Can you work these out from the model? Positions are in its coordinate system, mm. A direction names the side the tool comes from. Coordinates: 2 decimals unless noted, no trailing zeros. Loops run counter-clockwise (first coordinate to the right, second up) from the corner with the lowest first, then second, coordinate; pieces in that order, holes last. Notation, with made-up numbers: M 18,29 L 37,29 A9 cw 37,34 Z; hole C 82.5,28 d10. An arc over 180 degrees is marked long. Answer as a JSON object with one key per item and string values. Group by question number.
Item 1: We'd pull the mould along Y, two halves only. Please class faces 5 (the flat face through (-2, -12.5, 5)), 6 (the flat face through (-126, 91.5, 5)), 7 (the flat face through (-2, 86, 0)), 8 (the flat face through (126, -0.5, 5)): +Y half, -Y half, draft (parallel to the pull), parting line (faces both ways), or undercut.
Item 2: Suppose I cut it at C-C (z = 5). Count the separate pieces of the cut face and the enclosed holes in it, then the cut area to 3 significant figures.
Item 3: Suppose I cut it at A-A (x = 89). Write out the boundary of the cut face in (y, z).
Item 4: If I drill on line 1 (Y direction, x = -65, z = 4); line 2 (X direction, y = 67, z = 4); line 3 (Y direction, x = -35.5, z = 9.75), over which ranges is the centre line in solid material (lowest first)?
Item 5: I'm going to push flat-ended pins straight in: pin 1 Ø1.5 at (x, y) = (-18.5, 9) entering from -Z; pin 2 Ø1.5 at (y, z) = (51.5, 6.5) entering from +X; pin 3 Ø3 at (y, z) = (27.5, 6.5) entering from -X; pin 4 Ø5 at (x, z) = (-128.97, 5) entering from -Y. Where does each tip first touch, or does it pass through?
Item 6: Suppose I cut it at B-B (y = 36.5). Write out the boundary of the cut face in (x, z).
Item 7: Which directions (+Z, -Z, +X, -X, +Y, -Y) give clear straight access to the entire face, cutting with the end or side of a thin tool? Please do faces 1 (the flat face through (-126, -0.5, 5)), 2 (the flat face through (-132.966, 89, 5)), 3 (the cylindrical face through (-115.066, 79.546, 4.93)), 4 (the flat face through (109, 94, 2)).
```python
from build123d import *

# Parameters (mm, degrees)
SKETCH_1_R          = 5
SKETCH_1_W          = 100
SKETCH_1_H          = 77
EXTRUDE_1_DEPTH     = 10
SKETCH_3_R          = 7.5
CUT_EXTRUDE_1_DEPTH = 8
CUT_EXTRUDE_2_REACH = 166.385
SKETCH_5_R          = 2
SKETCH_6_W          = 8
SKETCH_6_H          = 12
EXTRUDE_2_DEPTH     = 10
SKETCH_7_W          = 15
SKETCH_7_H          = 1
CUT_EXTRUDE_3_DEPTH = 170.411241918
SKETCH_8_R          = 2
CUT_EXTRUDE_4_DEPTH = 174.176698457
SKETCH_9_R          = 4.5
CUT_EXTRUDE_5_DEPTH = 10
CHAMFER_1_SIZE      = 2


with BuildPart() as part:
    # 草图1 → 凸台-拉伸1 (new body)
    with BuildSketch(Plane.XY):
        with BuildLine():
            Line((-104, 84.5), (-70, 84.5))
            Line((-70, 84.5), (-70, 7.5))
            Line((-70, 7.5), (-104, 7.5))
            ThreePointArc((-104, 7.5), (-125.180339887, 5.590169944), (-114, -12.5))
            Line((-114, -12.5), (114, -12.5))
            ThreePointArc((114, -12.5), (125.180339887, 5.590169944), (104, 7.5))
            Line((104, 7.5), (70, 7.5))
            Line((70, 7.5), (70, 84.5))
            Line((70, 84.5), (104, 84.5))
            ThreePointArc((104, 84.5), (125.180339887, 86.409830056), (114, 104.5))
            Line((114, 104.5), (64, 104.5))
            Line((64, 104.5), (-64, 104.5))
            Line((-64, 104.5), (-114, 104.5))
            ThreePointArc((-114, 104.5), (-125.180339887, 86.409830056), (-104, 84.5))
        make_face()
        with Locations((-114, 0)):
            Circle(SKETCH_1_R, mode=Mode.SUBTRACT)
        with Locations((-114, 92)):
            Circle(SKETCH_1_R, mode=Mode.SUBTRACT)
        with Locations(Location((114, 92, 0), (0, 0, 180))):
            Circle(SKETCH_1_R, mode=Mode.SUBTRACT)
        with Locations(Location((114, 0, 0), (0, 0, 180))):
            Circle(SKETCH_1_R, mode=Mode.SUBTRACT)
        with Locations((0, 46)):
            Rectangle(SKETCH_1_W, SKETCH_1_H, mode=Mode.SUBTRACT)
    extrude(amount=EXTRUDE_1_DEPTH)

    # 草图3 → 切除-拉伸1 (cut)
    with BuildSketch(Plane.XY.offset(10)):
        with Locations((-114, 92)):
            Circle(SKETCH_3_R)
        with Locations((-114, 0)):
            Circle(SKETCH_3_R)
        with Locations(Location((114, 0, 0), (0, 0, 180))):
            Circle(SKETCH_3_R)
        with Locations(Location((114, 92, 0), (0, 0, 180))):
            Circle(SKETCH_3_R)
    extrude(amount=-CUT_EXTRUDE_1_DEPTH, mode=Mode.SUBTRACT)

    # 草图5 → 切除-拉伸2 (cut, up to next)
    with BuildSketch(Plane.XY, mode=Mode.PRIVATE) as cut_extrude_2_sk1:
        with Locations(Location((-65, 94.5, 0), (0, 0, 180))):
            Circle(SKETCH_5_R)
    cut_extrude_2_tool1 = extrude(cut_extrude_2_sk1.sketch, amount=CUT_EXTRUDE_2_REACH, mode=Mode.PRIVATE) & part.part
    # 草图5 → 切除-拉伸2 (cut, up to next)
    with BuildSketch(Plane.XY, mode=Mode.PRIVATE) as cut_extrude_2_sk2:
        with Locations(Location((-75, 94.5, 0), (0, 0, 180))):
            Circle(SKETCH_5_R)
    cut_extrude_2_tool2 = extrude(cut_extrude_2_sk2.sketch, amount=CUT_EXTRUDE_2_REACH, mode=Mode.PRIVATE) & part.part
    # 草图5 → 切除-拉伸2 (cut, up to next)
    with BuildSketch(Plane.XY, mode=Mode.PRIVATE) as cut_extrude_2_sk3:
        with Locations(Location((-65, 69.5, 0), (0, 0, 180))):
            Circle(SKETCH_5_R)
    cut_extrude_2_tool3 = extrude(cut_extrude_2_sk3.sketch, amount=CUT_EXTRUDE_2_REACH, mode=Mode.PRIVATE) & part.part
    # 草图5 → 切除-拉伸2 (cut, up to next)
    with BuildSketch(Plane.XY, mode=Mode.PRIVATE) as cut_extrude_2_sk4:
        with Locations(Location((-65, 22.5, 0), (0, 0, 180))):
            Circle(SKETCH_5_R)
    cut_extrude_2_tool4 = extrude(cut_extrude_2_sk4.sketch, amount=CUT_EXTRUDE_2_REACH, mode=Mode.PRIVATE) & part.part
    # 草图5 → 切除-拉伸2 (cut, up to next)
    with BuildSketch(Plane.XY, mode=Mode.PRIVATE) as cut_extrude_2_sk5:
        with Locations(Location((-65, -2.5, 0), (0, 0, 180))):
            Circle(SKETCH_5_R)
    cut_extrude_2_tool5 = extrude(cut_extrude_2_sk5.sketch, amount=CUT_EXTRUDE_2_REACH, mode=Mode.PRIVATE) & part.part
    # 草图5 → 切除-拉伸2 (cut, up to next)
    with BuildSketch(Plane.XY, mode=Mode.PRIVATE) as cut_extrude_2_sk6:
        with Locations(Location((-75, -2.5, 0), (0, 0, 180))):
            Circle(SKETCH_5_R)
    cut_extrude_2_tool6 = extrude(cut_extrude_2_sk6.sketch, amount=CUT_EXTRUDE_2_REACH, mode=Mode.PRIVATE) & part.part
    # 草图5 → 切除-拉伸2 (cut, up to next)
    with BuildSketch(Plane.XY, mode=Mode.PRIVATE) as cut_extrude_2_sk7:
        with Locations(Location((75, -2.5, 0), (0, 0, 180))):
            Circle(SKETCH_5_R)
    cut_extrude_2_tool7 = extrude(cut_extrude_2_sk7.sketch, amount=CUT_EXTRUDE_2_REACH, mode=Mode.PRIVATE) & part.part
    # 草图5 → 切除-拉伸2 (cut, up to next)
    with BuildSketch(Plane.XY, mode=Mode.PRIVATE) as cut_extrude_2_sk8:
        with Locations(Location((65, -2.5, 0), (0, 0, 180))):
            Circle(SKETCH_5_R)
    cut_extrude_2_tool8 = extrude(cut_extrude_2_sk8.sketch, amount=CUT_EXTRUDE_2_REACH, mode=Mode.PRIVATE) & part.part
    # 草图5 → 切除-拉伸2 (cut, up to next)
    with BuildSketch(Plane.XY, mode=Mode.PRIVATE) as cut_extrude_2_sk9:
        with Locations(Location((65, 22.5, 0), (0, 0, 180))):
            Circle(SKETCH_5_R)
    cut_extrude_2_tool9 = extrude(cut_extrude_2_sk9.sketch, amount=CUT_EXTRUDE_2_REACH, mode=Mode.PRIVATE) & part.part
    # 草图5 → 切除-拉伸2 (cut, up to next)
    with BuildSketch(Plane.XY, mode=Mode.PRIVATE) as cut_extrude_2_sk10:
        with Locations(Location((65, 69.5, 0), (0, 0, 180))):
            Circle(SKETCH_5_R)
    cut_extrude_2_tool10 = extrude(cut_extrude_2_sk10.sketch, amount=CUT_EXTRUDE_2_REACH, mode=Mode.PRIVATE) & part.part
    # 草图5 → 切除-拉伸2 (cut, up to next)
    with BuildSketch(Plane.XY, mode=Mode.PRIVATE) as cut_extrude_2_sk11:
        with Locations(Location((75, 94.5, 0), (0, 0, 180))):
            Circle(SKETCH_5_R)
    cut_extrude_2_tool11 = extrude(cut_extrude_2_sk11.sketch, amount=CUT_EXTRUDE_2_REACH, mode=Mode.PRIVATE) & part.part
    # 草图5 → 切除-拉伸2 (cut, up to next)
    with BuildSketch(Plane.XY, mode=Mode.PRIVATE) as cut_extrude_2_sk12:
        with Locations(Location((65, 94.5, 0), (0, 0, 180))):
            Circle(SKETCH_5_R)
    cut_extrude_2_tool12 = extrude(cut_extrude_2_sk12.sketch, amount=CUT_EXTRUDE_2_REACH, mode=Mode.PRIVATE) & part.part
    add(cut_extrude_2_tool1.solids().sort_by_distance((-65, 94.5, 0))[0], mode=Mode.SUBTRACT)
    add(cut_extrude_2_tool2.solids().sort_by_distance((-75, 94.5, 0))[0], mode=Mode.SUBTRACT)
    add(cut_extrude_2_tool3.solids().sort_by_distance((-65, 69.5, 0))[0], mode=Mode.SUBTRACT)
    add(cut_extrude_2_tool4.solids().sort_by_distance((-65, 22.5, 0))[0], mode=Mode.SUBTRACT)
    add(cut_extrude_2_tool5.solids().sort_by_distance((-65, -2.5, 0))[0], mode=Mode.SUBTRACT)
    add(cut_extrude_2_tool6.solids().sort_by_distance((-75, -2.5, 0))[0], mode=Mode.SUBTRACT)
    add(cut_extrude_2_tool7.solids().sort_by_distance((75, -2.5, 0))[0], mode=Mode.SUBTRACT)
    add(cut_extrude_2_tool8.solids().sort_by_distance((65, -2.5, 0))[0], mode=Mode.SUBTRACT)
    add(cut_extrude_2_tool9.solids().sort_by_distance((65, 22.5, 0))[0], mode=Mode.SUBTRACT)
    add(cut_extrude_2_tool10.solids().sort_by_distance((65, 69.5, 0))[0], mode=Mode.SUBTRACT)
    add(cut_extrude_2_tool11.solids().sort_by_distance((75, 94.5, 0))[0], mode=Mode.SUBTRACT)
    add(cut_extrude_2_tool12.solids().sort_by_distance((65, 94.5, 0))[0], mode=Mode.SUBTRACT)

    # 草图6 → 凸台-拉伸2 (add)
    with BuildSketch(Plane.XY.offset(10)):
        with Locations((128.9658561, 92)):
            Rectangle(SKETCH_6_W, SKETCH_6_H)
        with Locations((128.9658561, 0)):
            Rectangle(SKETCH_6_W, SKETCH_6_H)
        with Locations((-128.9658561, 0)):
            Rectangle(SKETCH_6_W, SKETCH_6_H)
        with Locations((-128.9658561, 92)):
            Rectangle(SKETCH_6_W, SKETCH_6_H)
    extrude(amount=-EXTRUDE_2_DEPTH)

    # 草图7 → 切除-拉伸3 (cut, through all)
    with BuildSketch(Plane.XY.offset(10)):
        with Locations((125.4658561, 92)):
            Rectangle(SKETCH_7_W, SKETCH_7_H)
        with Locations((125.4658561, 0)):
            Rectangle(SKETCH_7_W, SKETCH_7_H)
        with Locations((-125.4658561, 0)):
            Rectangle(SKETCH_7_W, SKETCH_7_H)
        with Locations((-125.4658561, 92)):
            Rectangle(SKETCH_7_W, SKETCH_7_H)
    extrude(amount=-CUT_EXTRUDE_3_DEPTH, mode=Mode.SUBTRACT)

    # 草图8 → 切除-拉伸4 (cut, through all)
    with BuildSketch(Plane(origin=(0, 98, 0), x_dir=(1, 0, 0), z_dir=(0, 1, 0))):
        with Locations(Location((-128.9658561, -5, 0), (0, 0, 180))):
            Circle(SKETCH_8_R)
        with Locations(Location((128.9658561, -5, 0), (0, 0, 90))):
            Circle(SKETCH_8_R)
    extrude(amount=-CUT_EXTRUDE_4_DEPTH, mode=Mode.SUBTRACT)

    # 草图9 → 切除-拉伸5 (cut)
    with BuildSketch(Plane(origin=(0, 98, 0), x_dir=(1, 0, 0), z_dir=(0, 1, 0))):
        with Locations((-128.9658561, -5)):
            Circle(SKETCH_9_R)
        with Locations((128.9658561, -5)):
            Circle(SKETCH_9_R)
    extrude(amount=CUT_EXTRUDE_5_DEPTH, mode=Mode.SUBTRACT)

    # 倒角1
    chamfer_1_edges = [part.edges().sort_by_distance(p)[0] for p in [
        (-73, -2.5, 0),
        (77, -2.5, 0),
        (67, -2.5, 0),
        (67, 22.5, 0),
        (-63, -2.5, 0),
        (-63, 22.5, 0),
        (-63, 69.5, 0),
        (-73, 94.5, 0),
        (67, 94.5, 0),
        (77, 94.5, 0),
        (67, 69.5, 0),
        (-63, 94.5, 0),
    ]]
    chamfer(chamfer_1_edges, length=CHAMFER_1_SIZE)


solid = part.part
```
From the geometry:
{
 "1": {"face 5": "-Y half", "face 6": "undercut", "face 7": "draft", "face 8": "undercut"},
 "2": {"separate pieces": "9", "enclosed holes": "13", "area": "12,600 mm2"},
 "3": {"outline": "M -12.5,0 L 7.5,0 L 7.5,10 L -12.5,10 Z; M 84.5,0 L 104.5,0 L 104.5,10 L 84.5,10 Z"},
 "4": {"line 1": "-12.5 to -4.5, -0.5 to 20.5, 24.5 to 67.5, 71.5 to 92.5, 96.5 to 104.5", "line 2": "-70 to -50, 50 to 70", "line 3": "-12.5 to 7.5, 84.5 to 104.5"},
 "5": {"pin 1": "through", "pin 2": "x = 70", "pin 3": "x = -70", "pin 4": "y = -6"},
 "6": {"outline": "M -70,0 L -50,0 L -50,10 L -70,10 Z; M 50,0 L 70,0 L 70,10 L 50,10 Z"},
 "7": {"face 1": "+Z, -Z, -X", "face 2": "+Z, -Z, -X, +Y, -Y", "face 3": "+Z, -Z", "face 4": "+Z"}
}
